```python
from build123d import *

# Parameters (mm, degrees)
BOSS_EXTRU_1_DEPTH      = 8.1
ESQUISSE2_R             = 1.65
ENL_V_MAT_EXTRU_1_DEPTH = 142.653132687


with BuildPart() as part:
    # Esquisse1 → Boss.-Extru.1 (new body)
    with BuildSketch(Plane.XY):
        Polygon((0, 0), (0, 20), (8, 20), (10, 22), (10, 118), (8, 120), (0, 120), (0, 140), (2.142135624, 140), (20, 122.142135624), (20, 17.857864376), (2.142135624, 0), align=None)
    extrude(amount=BOSS_EXTRU_1_DEPTH)

    # Esquisse2 → Enlèv. mat.-Extru.1 (cut, through all)
    with BuildSketch(Plane.ZY):
        with Locations((4.05, 15)):
            Circle(ESQUISSE2_R)
        with Locations(Location((4.05, 5, 0), (0, 0, 270))):
            Circle(ESQUISSE2_R)
        with Locations((4.05, 135)):
            Circle(ESQUISSE2_R)
        with Locations(Location((4.05, 125, 0), (0, 0, 90))):
            Circle(ESQUISSE2_R)
    extrude(amount=-ENL_V_MAT_EXTRU_1_DEPTH, mode=Mode.SUBTRACT)


solid = part.part
```
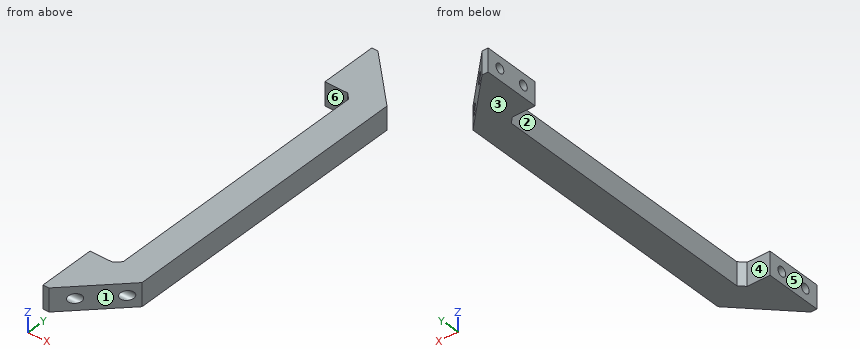
Geometry check sheet. Reference: the model listing, model coordinates, mm. Face numbers are marked on the shaded views. A direction names the side the tool comes from. Coordinates: 2 decimals unless noted, no trailing zeros. Order: outer loops, then holes, each group sorted by start corner. A loop starts at its lowest first (then second) coordinate and runs counter-clockwise, first axis right, second up. Notation, with made-up numbers: (66.5, -34.75) - (104.5, -34.75) arc R14 cw to (104.5, -16.75) - close; hole circle Ø4 at (81.5, 35.25). An arc over 180 degrees is marked (long way). Use one line per item in the form item = value.
1. Scan lines: line 1 (Z direction, x = 6.75, y = 5); line 2 (Y direction, x = 3.75, z = 4.05); line 3 (Y direction, x = 1.5, z = 2). Record each from-to range of solid material in increasing order.
Here are the results:
line_1 = 0 to 2.4, 5.7 to 8.1
line_2 = 1.61 to 3.35, 6.65 to 13.35, 16.65 to 20, 120 to 123.35, 126.65 to 133.35, 136.65 to 138.39
line_3 = 0 to 20, 120 to 140
2. Access from +Z, -Z, +X, -X, +Y, -Y to the whole of each face (thin tool, end or side, straight path). Record for the marked faces 5 and 6.
Here are the results:
face_5 = +Z, -Z, -X, +Y, -Y
face_6 = +Z, -Z, -X
3. Section check A-A (y = 5). Record the boundary of the cut face in (x, z), then the cut area to 3 significant figures.
Here are the results:
outline = (0, 0) - (7.14, 0) - (7.14, 2.4) - (0, 2.4) - close; (0, 5.7) - (7.14, 5.7) - (7.14, 8.1) - (0, 8.1) - close
area = 34.3 mm²
4. Gauge pin test, flat ends, axial feed: pin 1 (1 mm diameter, centred on x = 13.5, z = 1, fed in from +Y); pin 2 (2 mm diameter, centred on x = 6, z = 6.5, fed in from +Y); pin 3 (4 mm diameter, centred on x = 5, z = 5, fed in from +Y). Record the tip position at first contact, or that the pin passes through.
Here are the results:
pin_1 = 129.14
pin_2 = 137.14
pin_3 = 139.14
5. Draft check along Y on the marked faces 1, 2, 3 and 4. Enter one of: pulls with the +Y half, pulls with the -Y half, needs draft (parallel to the pull), parting line crosses it, or undercut.
Here are the results:
face_1 = pulls with the -Y half
face_2 = undercut
face_3 = needs draft
face_4 = undercut
6. Section check B-B (y = 113.5). Record the boundary of the cut face in (x, z).
Here are the results:
outline = (10, 0) - (20, 0) - (20, 8.1) - (10, 8.1) - close
